Input: dimensioned drawing with shaded views. Units: mm. Origin: part minimum x, y, z. Coordinates: 2 decimals unless noted, no trailing zeros. Write each loop counter-clockwise with the first axis right and the second up, starting at its lowest first coordinate (ties: lowest second). Pieces come first, ordered by that corner, then holes. Notation, with made-up numbers: M 3.5,-8 L 41.5,-8 A21 ccw 41.5,13 Z; hole C -38.75,72.25 d2. An arc over 180 degrees is marked long. Use one line per item in the form item = value.
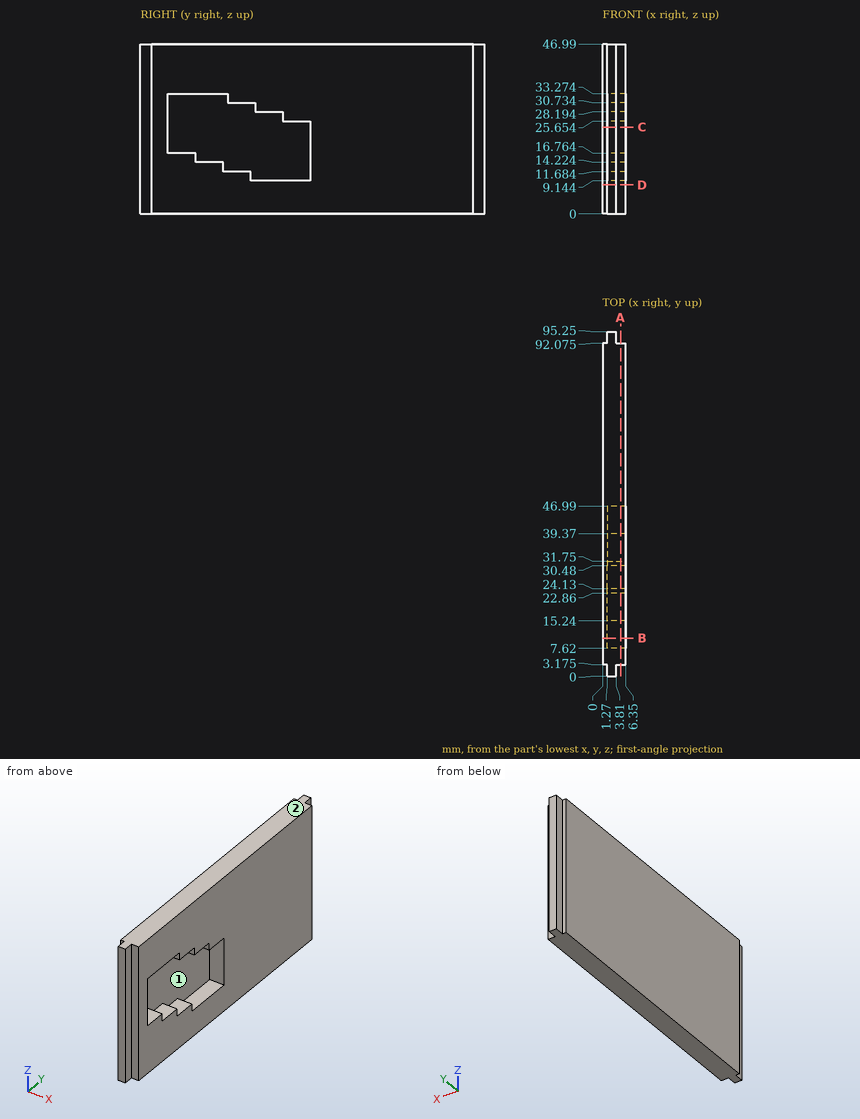
(1) Section query C-C on z = 24. Return the cut outline in (x, y) (3 decimals).
Computed:
outline = M 0,3.175 L 1.27,3.175 L 1.27,0 L 3.81,0 L 3.81,3.175 L 6.35,3.175 L 6.35,7.62 L 1.27,7.62 L 1.27,46.99 L 6.35,46.99 L 6.35,92.075 L 3.81,92.075 L 3.81,95.25 L 1.27,95.25 L 1.27,92.075 L 0,92.075 Z
(2) Section query B-B on y = 10.5. Return the cut outline in (x, z), plus the area to 3 significant figures.
Computed:
outline = M 0,0 L 6.35,0 L 6.35,16.76 L 1.27,16.76 L 1.27,33.27 L 6.35,33.27 L 6.35,46.99 L 0,46.99 Z
area = 215 mm^2
(3) Pull-direction query (Y, two-part tool) for the marked faces 1 and 2; classes: pulls with the +Y half, pulls with the -Y half, needs draft (parallel to the pull), parting line crosses it, or undercut.
Computed:
face_1 = undercut
face_2 = needs draft
(4) First-contact query: pin 1 Ø1 at (x, z) = (0.5, 14) entering from -Y (3 decimals); pin 2 Ø1.3 at (x, z) = (5, 27) entering from +Y (3 decimals); pin 3 Ø3.5 at (y, z) = (94, 17) entering from -X. Flat tips, straight axial feed; report the tip coordinate or a pass-through.
Computed:
pin_1 = 3.175
pin_2 = 92.075
pin_3 = 1.27
(5) Line query: probe 1 along Z at (x, y) = (3.75, 26); probe 2 along Z at (x, y) = (5.75, 35); probe 3 along Y at (x, z) = (4.5, 20) (3 decimals). Output: solid intervals per line, ascending.
Computed:
probe_1 = 0 to 11.68, 30.73 to 46.99
probe_2 = 0 to 9.14, 28.19 to 46.99
probe_3 = 3.175 to 7.62, 46.99 to 92.075
(6) Section query D-D on z = 8. Return the cut outline in (x, y) (3 decimals), plus the area to 3 significant figures.
Computed:
outline = M 0,3.175 L 1.27,3.175 L 1.27,0 L 3.81,0 L 3.81,3.175 L 6.35,3.175 L 6.35,92.075 L 3.81,92.075 L 3.81,95.25 L 1.27,95.25 L 1.27,92.075 L 0,92.075 Z
area = 581 mm^2
(7) Section query A-A on x = 5. Return the cut outline in (y, z) (3 decimals), plus the area to 3 significant figures.
Computed:
outline = M 3.175,0 L 92.075,0 L 92.075,46.99 L 3.175,46.99 Z; hole M 7.62,16.764 L 15.24,16.764 L 15.24,14.224 L 22.86,14.224 L 22.86,11.684 L 30.48,11.684 L 30.48,9.144 L 46.99,9.144 L 46.99,25.654 L 39.37,25.654 L 39.37,28.194 L 31.75,28.194 L 31.75,30.734 L 24.13,30.734 L 24.13,33.274 L 7.62,33.274 Z
area = 3,460 mm^2
